Source: CAD feature listing. Evaluate the final solid. Frame: model axes, mm. Round coordinates to 2 decimals unless told otherwise and drop trailing zeros. Write each loop counter-clockwise with the first axis right and the second up, starting at its lowest first coordinate (ties: lowest second). Pieces come first, ordered by that corner, then holes. Notation, with made-up numbers: M 74.5,-27.75 L 92.5,-27.75 A12 ccw 92.5,-6.75 Z; hole C 78.25,-5 d8. An arc over 180 degrees is marked long. Answer in a Markdown table with one row per item. Add a question column.
Item 1: Material intervals for probe 1 along Z at (x, y) = (29.5, 0.75); probe 2 along X at (y, z) = (0.4, 11.5); probe 3 along X at (y, z) = (1, -12), sorted ascending.
Item 2: Cut plane B-B on z = 47. Return loops of the section in (x, y), and give its area (3 significant figures).
Item 3: Contact query for flat-ended pins moving along their axis: pin 1 (1 mm diameter, centred on x = 84, z = -27, fed in from -Y); pin 2 (3.5 mm diameter, centred on x = 167.89, z = -117.12, fed in from -Y). Output: stop coordinate, or through.
Item 4: Cut plane A-A on x = -24. Return loops of the section in (y, z), and give its area (3 significant figures).
Item 5: Cut plane C-C on y = 0.7. Give the number of separate pieces and of enclosed holes in the cut face, and give its area (3 significant figures).
from build123d import *

# Parameters (mm, degrees)
SKETCH_1_W          = 330
SKETCH_1_H          = 225
EXTRUDE_1_DEPTH     = 3
SKETCH_3_R          = 2
CUT_EXTRUDE_1_DEPTH = 225.719219269
CUT_EXTRUDE_2_DEPTH = 225.719219269
CUT_EXTRUDE_3_DEPTH = 225.719219269
CUT_EXTRUDE_4_DEPTH = 225.719219269


with BuildPart() as part:
    # 草图1 → 凸台-拉伸1 (new body)
    with BuildSketch(Plane(origin=(0, 0, 0), x_dir=(1, 0, 0), z_dir=(0, 1, 0))):
        with Locations((19.411764706, 15.882352941)):
            Rectangle(SKETCH_1_W, SKETCH_1_H)
    extrude(amount=EXTRUDE_1_DEPTH)

    # 草图3 → 切除-拉伸1 (cut, through all)
    with BuildSketch(Plane(origin=(0, 3, 0), x_dir=(1, 0, 0), z_dir=(0, 1, 0))):
        with Locations(Location((-129.063688438, 117.115616448, 0), (0, 0, 270))):
            Circle(SKETCH_3_R)
        with Locations(Location((167.88721785, 117.115616448, 0), (0, 0, 90))):
            Circle(SKETCH_3_R)
        with Locations(Location((-60.588235294, -86.617647059, 0), (0, 0, 270))):
            Circle(SKETCH_3_R)
        with Locations(Location((99.411764706, -86.617647059, 0), (0, 0, 90))):
            Circle(SKETCH_3_R)
    extrude(amount=-CUT_EXTRUDE_1_DEPTH, mode=Mode.SUBTRACT)

    # 草图4 → 切除-拉伸2 (cut, through all)
    with BuildSketch(Plane(origin=(0, 3, 0), x_dir=(1, 0, 0), z_dir=(0, 1, 0))):
        with BuildLine():
            Line((-116.235231271, -14.117647059), (-116.235231271, 45.882352941))
            ThreePointArc((-116.235231271, 45.882352941), (-111.235231271, 50.882352941), (-106.235231271, 45.882352941))
            Line((-106.235231271, 45.882352941), (-106.235231271, -14.117647059))
            ThreePointArc((-106.235231271, -14.117647059), (-111.235231271, -19.117647059), (-116.235231271, -14.117647059))
        make_face()
        with BuildLine():
            Line((155.058760683, -14.117647059), (155.058760683, 45.882352941))
            ThreePointArc((155.058760683, 45.882352941), (150.058760683, 50.882352941), (145.058760683, 45.882352941))
            Line((145.058760683, 45.882352941), (145.058760683, -14.117647059))
            ThreePointArc((145.058760683, -14.117647059), (150.058760683, -19.117647059), (155.058760683, -14.117647059))
        make_face()
    extrude(amount=-CUT_EXTRUDE_2_DEPTH, mode=Mode.SUBTRACT)

    # 草图5 → 切除-拉伸3 (cut, through all)
    with BuildSketch(Plane(origin=(0, 3, 0), x_dir=(1, 0, 0), z_dir=(0, 1, 0))):
        with BuildLine():
            Line((-74.774602087, 85.1003303), (113.598131499, 85.1003303))
            ThreePointArc((113.598131499, 85.1003303), (118.598131499, 80.1003303), (113.598131499, 75.1003303))
            Line((113.598131499, 75.1003303), (-74.774602087, 75.1003303))
            ThreePointArc((-74.774602087, 75.1003303), (-79.774602087, 80.1003303), (-74.774602087, 85.1003303))
        make_face()
        with BuildLine():
            Line((-74.774602087, -53.335624418), (113.598131499, -53.335624418))
            ThreePointArc((113.598131499, -53.335624418), (118.598131499, -48.335624418), (113.598131499, -43.335624418))
            Line((113.598131499, -43.335624418), (-74.774602087, -43.335624418))
            ThreePointArc((-74.774602087, -43.335624418), (-79.774602087, -48.335624418), (-74.774602087, -53.335624418))
        make_face()
    extrude(amount=-CUT_EXTRUDE_3_DEPTH, mode=Mode.SUBTRACT)

    # 草图6 → 切除-拉伸4 (cut, through all)
    with BuildSketch(Plane(origin=(0, 3, 0), x_dir=(1, 0, 0), z_dir=(0, 1, 0))):
        with BuildLine():
            Line((-74.773235294, 20.882352941), (113.596764706, 20.882352941))
            ThreePointArc((113.596764706, 20.882352941), (118.596764706, 15.882352941), (113.596764706, 10.882352941))
            Line((113.596764706, 10.882352941), (-74.773235294, 10.882352941))
            ThreePointArc((-74.773235294, 10.882352941), (-79.773235294, 15.882352941), (-74.773235294, 20.882352941))
        make_face()
    extrude(amount=-CUT_EXTRUDE_4_DEPTH, mode=Mode.SUBTRACT)


solid = part.part
Results below:
| question | item | result |
|---|---|---|
| 1 | probe 1 | -128.38 to -85.1, -75.1 to -20.88, -10.88 to 43.34, 53.34 to 96.62 |
| 1 | probe 2 | -145.59 to -116.24, -106.24 to 145.06, 155.06 to 184.41 |
| 1 | probe 3 | -145.59 to -116.24, -106.24 to -77.92, 116.75 to 145.06, 155.06 to 184.41 |
| 2 | outline | M -145.59,0 L -79.59,0 L -79.59,3 L -145.59,3 Z; M 118.42,0 L 184.41,0 L 184.41,3 L 118.42,3 Z |
| 2 | area | 396 mm2 |
| 3 | pin 1 | y = 0 |
| 3 | pin 2 | through |
| 4 | outline | M 0,-128.38 L 3,-128.38 L 3,-85.1 L 0,-85.1 Z; M 0,-75.1 L 3,-75.1 L 3,-20.88 L 0,-20.88 Z; M 0,-10.88 L 3,-10.88 L 3,43.34 L 0,43.34 Z; M 0,53.34 L 3,53.34 L 3,96.62 L 0,96.62 Z |
| 4 | area | 585 mm2 |
| 5 | separate pieces | 1 |
| 5 | enclosed holes | 9 |
| 5 | area | 67,000 mm2 |
